For this review, take the finished solid that the model builds, in its own axes (mm). Round coordinates to 2 decimals unless told otherwise and drop trailing zeros. Order: outer loops, then holes, each group sorted by start corner. A loop starts at its lowest first (then second) coordinate and runs counter-clockwise, first axis right, second up. Notation, with made-up numbers: (71, 15.5) -> (86, 15.5) arc R21 cw to (86, 52.5) -> close; hole circle Ø8 at (23.5, 75). An arc over 180 degrees is marked (long way). Use a Markdown table: item, result. Add a question column.
1) Consider section B-B (z = 1.5). State the section outline as (x, y) points, plus the area to 3 significant figures.
2) Draft analysis for pull direction X (two halves, no side actions). For faces 1 (the face through (7.434, 34.466, 3.219)), 2 (the face through (38.1, 23, 3)), 3 (the face through (19, 23, 6.35)), state which applies: pulls with the +X half, pulls with the -X half, needs draft (parallel to the pull), parting line crosses it, or undercut.
3) Wall thickness on line 1 along Y through (x, z) = (11.43, 5); line 2 along Y through (x, z) = (13.5, 4.5); line 3 along X through (y, z) = (31, 6): over which ranges is each line inside the solid? List them lowest first. Write a range as [from, to].
4) Consider section A-A (x = 11.43). State the section outline as (y, z) points.
5) Consider section C-C (y = 34.29). State the section outline as (x, z) points, plus the area to 3 significant figures.
```python
from build123d import *

# Parameters (mm, degrees)
SKETCH1_W               = 38.1
SKETCH1_H               = 45.72
BOSS_EXTRUDE1_DEPTH     = 6.35
SKETCH2_R               = 4
CUT_EXTRUDE1_DEPTH      = 1
CUT_EXTRUDE1_DEPTH_BACK = 7.35


with BuildPart() as part:
    # Sketch1 → Boss-Extrude1 (new body)
    with BuildSketch(Plane.XY):
        with Locations((19.05, 22.86)):
            Rectangle(SKETCH1_W, SKETCH1_H)
    extrude(amount=BOSS_EXTRUDE1_DEPTH)

    # Sketch2 → Cut-Extrude1 (cut, two sides)
    with BuildSketch(Plane.XY.offset(6.35)) as cut_extrude1_sk:
        with Locations((11.43, 34.29)):
            Circle(SKETCH2_R)
    extrude(amount=CUT_EXTRUDE1_DEPTH, mode=Mode.SUBTRACT)
    extrude(cut_extrude1_sk.sketch, amount=-CUT_EXTRUDE1_DEPTH_BACK, mode=Mode.SUBTRACT)


solid = part.part
```
Results list:
| question | item | result |
|---|---|---|
| 1 | outline | (0, 0) -> (38.1, 0) -> (38.1, 45.72) -> (0, 45.72) -> close; hole circle Ø8 at (11.43, 34.29) |
| 1 | area | 1,690 mm2 |
| 2 | face 1 | undercut |
| 2 | face 2 | pulls with the +X half |
| 2 | face 3 | needs draft |
| 3 | line 1 | [0, 30.29], [38.29, 45.72] |
| 3 | line 2 | [0, 30.87], [37.71, 45.72] |
| 3 | line 3 | [0, 9.15], [13.71, 38.1] |
| 4 | outline | (0, 0) -> (30.29, 0) -> (30.29, 6.35) -> (0, 6.35) -> close; (38.29, 0) -> (45.72, 0) -> (45.72, 6.35) -> (38.29, 6.35) -> close |
| 5 | outline | (0, 0) -> (7.43, 0) -> (7.43, 6.35) -> (0, 6.35) -> close; (15.43, 0) -> (38.1, 0) -> (38.1, 6.35) -> (15.43, 6.35) -> close |
| 5 | area | 191 mm2 |
